```python
from build123d import *

# Parameters (mm, degrees)
F1_DEPTH = 25.4
F2_DEPTH = 0.254
F3_R     = 3.175
F4_DEPTH = 0.254


with BuildPart() as f1:
    # F0 (on Front) → F1 (new body)
    with BuildSketch(Plane.XZ):
        with BuildLine():
            Line((-115.57, -153.67), (115.57, -153.67))
            ThreePointArc((115.57, -153.67), (120.060128, -151.810128), (121.92, -147.32))
            Line((121.92, -147.32), (121.92, 147.32))
            ThreePointArc((121.92, 147.32), (120.060128, 151.810128), (115.57, 153.67))
            Line((115.57, 153.67), (-115.57, 153.67))
            ThreePointArc((-115.57, 153.67), (-120.060128, 151.810128), (-121.92, 147.32))
            Line((-121.92, 147.32), (-121.92, -147.32))
            ThreePointArc((-121.92, -147.32), (-120.060128, -151.810128), (-115.57, -153.67))
        make_face()
        with BuildLine():
            ThreePointArc((120.65, -146.05), (118.790128, -150.540128), (114.3, -152.4))
            Line((114.3, -152.4), (-114.3, -152.4))
            ThreePointArc((-114.3, -152.4), (-118.790128, -150.540128), (-120.65, -146.05))
            Line((-120.65, -146.05), (-120.65, 146.05))
            ThreePointArc((-120.65, 146.05), (-118.790128, 150.540128), (-114.3, 152.4))
            Line((-114.3, 152.4), (114.3, 152.4))
            ThreePointArc((114.3, 152.4), (118.790128, 150.540128), (120.65, 146.05))
            Line((120.65, 146.05), (120.65, -146.05))
        make_face(mode=Mode.SUBTRACT)
    extrude(amount=F1_DEPTH)

    # F0 (on Front) → F2 (join)
    with BuildSketch(Plane.XZ):
        with BuildLine():
            Line((-114.3, -152.4), (114.3, -152.4))
            ThreePointArc((114.3, -152.4), (118.790128, -150.540128), (120.65, -146.05))
            Line((120.65, -146.05), (120.65, 146.05))
            ThreePointArc((120.65, 146.05), (118.790128, 150.540128), (114.3, 152.4))
            Line((114.3, 152.4), (-114.3, 152.4))
            ThreePointArc((-114.3, 152.4), (-118.790128, 150.540128), (-120.65, 146.05))
            Line((-120.65, 146.05), (-120.65, -146.05))
            ThreePointArc((-120.65, -146.05), (-118.790128, -150.540128), (-114.3, -152.4))
        make_face()
        with BuildLine():
            ThreePointArc((107.95, -133.35), (106.090128, -137.840128), (101.6, -139.7))
            Line((101.6, -139.7), (-101.6, -139.7))
            ThreePointArc((-101.6, -139.7), (-106.090128, -137.840128), (-107.95, -133.35))
            Line((-107.95, -133.35), (-107.95, 133.35))
            ThreePointArc((-107.95, 133.35), (-106.090128, 137.840128), (-101.6, 139.7))
            Line((-101.6, 139.7), (101.6, 139.7))
            ThreePointArc((101.6, 139.7), (106.090128, 137.840128), (107.95, 133.35))
            Line((107.95, 133.35), (107.95, -133.35))
        make_face(mode=Mode.SUBTRACT)
    extrude(amount=F2_DEPTH)

    # F3 (on face) → F4 (join)
    with BuildSketch(Plane.XZ.offset(25.4)):
        with BuildLine():
            Line((-121.92, 147.32), (-121.92, -147.32))
            ThreePointArc((-121.92, -147.32), (-120.060128, -151.810128), (-115.57, -153.67))
            Line((-115.57, -153.67), (115.57, -153.67))
            ThreePointArc((115.57, -153.67), (120.060128, -151.810128), (121.92, -147.32))
            Line((121.92, -147.32), (121.92, 147.32))
            ThreePointArc((121.92, 147.32), (120.060128, 151.810128), (115.57, 153.67))
            Line((115.57, 153.67), (-115.57, 153.67))
            ThreePointArc((-115.57, 153.67), (-120.060128, 151.810128), (-121.92, 147.32))
        make_face()
        with BuildLine():
            Line((120.65, 146.05), (120.65, -146.05))
            ThreePointArc((120.65, -146.05), (118.790128, -150.540128), (114.3, -152.4))
            Line((114.3, -152.4), (-114.3, -152.4))
            ThreePointArc((-114.3, -152.4), (-118.790128, -150.540128), (-120.65, -146.05))
            Line((-120.65, -146.05), (-120.65, 146.05))
            ThreePointArc((-120.65, 146.05), (-118.790128, 150.540128), (-114.3, 152.4))
            Line((-114.3, 152.4), (114.3, 152.4))
            ThreePointArc((114.3, 152.4), (118.790128, 150.540128), (120.65, 146.05))
        make_face(mode=Mode.SUBTRACT)
        with BuildLine():
            Line((-128.27, -165.1), (128.27, -165.1))
            ThreePointArc((128.27, -165.1), (132.760128, -163.240128), (134.62, -158.75))
            Line((134.62, -158.75), (134.62, 158.75))
            ThreePointArc((134.62, 158.75), (132.760128, 163.240128), (128.27, 165.1))
            Line((128.27, 165.1), (76.2, 165.1))
            Line((76.2, 165.1), (11.687881, 198.535574))
            ThreePointArc((11.687881, 198.535574), (0, 201.384445), (-11.687881, 198.535574))
            Line((-11.687881, 198.535574), (-76.2, 165.1))
            Line((-76.2, 165.1), (-128.27, 165.1))
            ThreePointArc((-128.27, 165.1), (-132.760128, 163.240128), (-134.62, 158.75))
            Line((-134.62, 158.75), (-134.62, -158.75))
            ThreePointArc((-134.62, -158.75), (-132.760128, -163.240128), (-128.27, -165.1))
        make_face()
        with Locations((-76.2, -158.75)):
            Circle(F3_R, mode=Mode.SUBTRACT)
        with Locations((0, -158.75)):
            Circle(F3_R, mode=Mode.SUBTRACT)
        with Locations((76.2, -158.75)):
            Circle(F3_R, mode=Mode.SUBTRACT)
        with BuildLine():
            ThreePointArc((-115.57, -153.67), (-120.060128, -151.810128), (-121.92, -147.32))
            Line((-121.92, -147.32), (-121.92, 147.32))
            ThreePointArc((-121.92, 147.32), (-120.060128, 151.810128), (-115.57, 153.67))
            Line((-115.57, 153.67), (115.57, 153.67))
            ThreePointArc((115.57, 153.67), (120.060128, 151.810128), (121.92, 147.32))
            Line((121.92, 147.32), (121.92, -147.32))
            ThreePointArc((121.92, -147.32), (120.060128, -151.810128), (115.57, -153.67))
            Line((115.57, -153.67), (-115.57, -153.67))
        make_face(mode=Mode.SUBTRACT)
        with Locations((-76.2, 158.75)):
            Circle(F3_R, mode=Mode.SUBTRACT)
        with Locations((0, 158.75)):
            Circle(F3_R, mode=Mode.SUBTRACT)
        with BuildLine():
            ThreePointArc((-3.81, 190.947112), (0, 194.757112), (3.81, 190.947112))
            Line((3.81, 190.947112), (11.45294, 190.947112))
            ThreePointArc((11.45294, 190.947112), (14.147017, 189.831189), (15.26294, 187.137112))
            ThreePointArc((15.26294, 187.137112), (14.147017, 184.443035), (11.45294, 183.327112))
            Line((11.45294, 183.327112), (-11.45294, 183.327112))
            ThreePointArc((-11.45294, 183.327112), (-15.26294, 187.137112), (-11.45294, 190.947112))
            Line((-11.45294, 190.947112), (-3.81, 190.947112))
        make_face(mode=Mode.SUBTRACT)
        with Locations((76.2, 158.75)):
            Circle(F3_R, mode=Mode.SUBTRACT)
    extrude(amount=-F4_DEPTH)


solid = f1.part
```
The listing builds one solid part. Answer for the finished solid, in the listing's coordinates (mm). A direction names the side the tool comes from. Give positions to 0.01 mm unless a question says otherwise; leave off trailing zeros. Write each loop counter-clockwise with the first axis right and the second up, starting at its lowest first coordinate (ties: lowest second). Pieces come first, ordered by that corner, then holes. Notation, with made-up numbers: (82, -2.75) - (135, -2.75) arc R30 ccw to (135, 30.25) - close; hole circle Ø8 at (-14, 3). An arc over 180 degrees is marked (long way). Use one line per item in the form item = value. Start each with the question number.
1) Flat-ended cylindrical pins translate along their axes: pin 1 Ø10 at (x, z) = (-4, 133) entering from +Y (3 decimals); pin 2 Ø1.5 at (x, y) = (-49, -10) entering from -Z; pin 3 Ø2 at (y, z) = (-5, 66.5) entering from +X. Find the tip coordinate at first contact, or state that the pin passes through.
2) The mould has two halves that part along Z. Classify faces 1 (the face through (121.92, -12, -2)), 2 (the face through (-2, -13, 152.4)), 3 (the face through (-2, -12, -153.67)): pulls with the +Z half, pulls with the -Z half, needs draft (parallel to the pull), parting line crosses it, or undercut.
3) Find section A-A on z = -121.5. Determine the outline of the cut face in (x, y).
4) Consider line 1 along X through (y, z) = (-25.3, 158.75) (3 decimals); line 2 along X through (y, z) = (-17.25, 112.5); line 3 along Z through (x, y) = (-31.5, -17.75). Determine where each line is inside the solid, lowest interval first. Write a range as from..to.
5) Find section B-B on y = -10. Determine the outline of the cut face in (x, z), plus the area to 3 significant figures.
6) A tool of negligible diameter and unlimited length cuts with its end or side. For faces 4 (the face through (2, -13, -152.4)), 5 (the face through (-130, -25.146, 19)), 6 (the face through (2, -12, 153.67)), from which of +Z, -Z, +X, -X, +Y, -Y can it reach the whole face along a straight path? Write none if from no direction.
7) Find section C-C on x = 20. Determine the outline of the cut face in (y, z).
Geometry results:
q1.pin_1 = through
q1.pin_2 = -153.67
q1.pin_3 = 121.92
q2.face_1 = needs draft
q2.face_2 = undercut
q2.face_3 = pulls with the -Z half
q3.outline = (-134.62, -25.4) - (-120.65, -25.4) - (-120.65, -0.25) - (-107.95, -0.25) - (-107.95, 0) - (-121.92, 0) - (-121.92, -25.15) - (-134.62, -25.15) - close; (107.95, -0.25) - (120.65, -0.25) - (120.65, -25.4) - (134.62, -25.4) - (134.62, -25.15) - (121.92, -25.15) - (121.92, 0) - (107.95, 0) - close
q4.line_1 = -134.62..-79.375, -73.025..-3.175, 3.175..73.025, 79.375..134.62
q4.line_2 = -121.92..-120.65, 120.65..121.92
q4.line_3 = -153.67..-152.4, 152.4..153.67
q5.outline = (-121.92, -147.32) arc R6.35 ccw to (-115.57, -153.67) - (115.57, -153.67) arc R6.35 ccw to (121.92, -147.32) - (121.92, 147.32) arc R6.35 ccw to (115.57, 153.67) - (-115.57, 153.67) arc R6.35 ccw to (-121.92, 147.32) - close; hole (-120.65, -146.05) arc R6.35 ccw to (-114.3, -152.4) - (114.3, -152.4) arc R6.35 ccw to (120.65, -146.05) - (120.65, 146.05) arc R6.35 ccw to (114.3, 152.4) - (-114.3, 152.4) arc R6.35 ccw to (-120.65, 146.05) - close
q5.area = 1,390 mm2
q6.face_4 = -Y
q6.face_5 = +Y
q6.face_6 = +Z, +X, -X, +Y
q7.outline = (-25.4, -165.1) - (-25.15, -165.1) - (-25.15, -153.67) - (0, -153.67) - (0, -139.7) - (-0.25, -139.7) - (-0.25, -152.4) - (-25.4, -152.4) - close; (-25.4, 152.4) - (-0.25, 152.4) - (-0.25, 139.7) - (0, 139.7) - (0, 153.67) - (-25.15, 153.67) - (-25.15, 194.23) - (-25.4, 194.23) - close
